The model under review builds one solid part; all positions refer to its coordinate system, in mm. A direction names the side the tool comes from. Round coordinates to 2 decimals unless told otherwise and drop trailing zeros. Write each loop counter-clockwise with the first axis right and the second up, starting at its lowest first coordinate (ties: lowest second). Pieces come first, ordered by that corner, then holes. Notation, with made-up numbers: M -26.75,21 L 12.25,21 A23 cw 12.25,41 Z; hole C 72.25,59.25 d5. An arc over 180 degrees is marked long. One line per item, written item: value. Start each with the question number.
1) Wall thickness on probe 1 along Y at (x, z) = (-6, 12); probe 2 along Z at (x, y) = (0, -1); probe 3 along Z at (x, y) = (0, 1.5): over which ranges is each line inside the solid? List them lowest first.
2) Tool access review of faces 4 (the face through (14.985, -2.218, -0.66)), 5 (the face through (2.2, 4.5, -11.2)): name each direction out of +Z, -Z, +X, -X, +Y, -Y from which nothing blocks a thin tool from reaching the whole face with its end or side.
3) For P1, Ø8, axis at y = -2.5, z = 5.5, coming from the +X side; P2, Ø4, axis at y = 7, z = 1.5, coming from the -X side; P3, Ø3, axis at y = 5.5, z = -6.5, coming from the -X side, all flat-tipped, find the tip position at first contact; note any pin that passes through.
4) Take a section at C-C, the plane z = 4. Write out the cut boundary in (x, y).
5) Take a section at D-D, the plane y = -1.5. Write out the cut boundary in (x, z), and give its area (3 significant figures).
6) Mouldability with a two-part tool opening along X and no side actions: class faces 1 (the face through (-2.2, 0, -11.2)), 2 (the face through (5.19, 2.22, 9.98)), 3 (the face through (0.65, 2.34, -1.01)) as +X half, -X half, draft (parallel to the pull), parting line (faces both ways), or undercut.
7) Take a section at A-A, the plane z = 0. Write out the cut boundary in (x, y).
8) Take a section at B-B, the plane x = 0. Write out the cut boundary in (y, z).
from build123d import *

# Parameters (mm, degrees)
SKETCH1_R            = 11.25
BOSS_EXTRUDE1_DEPTH  = 4.5
SKETCH2_R            = 15
BOSS_EXTRUDE2_DEPTH  = 4.5
SKETCH3_R            = 15
BOSS_EXTRUDE3_DEPTH  = 4.5
M2_CLEARANCE_HOLE1_D = 2.4


with BuildPart() as part:
    # Sketch1 → Boss-Extrude1 (new body)
    with BuildSketch(Plane(origin=(0, 0, 0), x_dir=(1, 0, 0), z_dir=(0, 1, 0))):
        Circle(SKETCH1_R)
    extrude(amount=BOSS_EXTRUDE1_DEPTH)

    # Sketch2 → Boss-Extrude2 (add)
    with BuildSketch(Plane(origin=(0, 4.5, 0), x_dir=(1, 0, 0), z_dir=(0, 1, 0))):
        Circle(SKETCH2_R)
    extrude(amount=BOSS_EXTRUDE2_DEPTH)

    # Sketch3 → Boss-Extrude3 (add)
    with BuildSketch(Plane(origin=(0, 0, 0), x_dir=(-1, 0, 0), z_dir=(0, -1, 0))):
        Circle(SKETCH3_R)
    extrude(amount=BOSS_EXTRUDE3_DEPTH)

    # M2 Clearance Hole1 (through all)
    with Locations(Plane(origin=(0, -4.5, 0), x_dir=(-1, 0, 0), z_dir=(0, -1, 0))):
        with Locations((0, 0)):
            Hole(M2_CLEARANCE_HOLE1_D / 2)


solid = part.part
Checked values:
1. probe 1: y = -4.5 to 0, 4.5 to 9
1. probe 2: z = -15 to -1.2, 1.2 to 15
1. probe 3: z = -11.25 to -1.2, 1.2 to 11.25
2. face 4: +Y, -Y
2. face 5: none
3. P1: stops at x = 14.92
3. P2: stops at x = -15
3. P3: stops at x = -14.14
4. outline: M -14.46,-4.5 L 14.46,-4.5 L 14.46,0 L 10.51,0 L 10.51,4.5 L 14.46,4.5 L 14.46,9 L -14.46,9 L -14.46,4.5 L -10.51,4.5 L -10.51,0 L -14.46,0 Z
5. outline: C 0,0 d30; hole C 0,0 d2.4
5. area: 702 mm2
6. face 1: draft
6. face 2: parting line
6. face 3: undercut
7. outline: M -15,-4.5 L -1.2,-4.5 L -1.2,9 L -15,9 L -15,4.5 L -11.25,4.5 L -11.25,0 L -15,0 Z; M 1.2,-4.5 L 15,-4.5 L 15,0 L 11.25,0 L 11.25,4.5 L 15,4.5 L 15,9 L 1.2,9 Z
8. outline: M -4.5,-15 L 0,-15 L 0,-11.25 L 4.5,-11.25 L 4.5,-15 L 9,-15 L 9,-1.2 L -4.5,-1.2 Z; M -4.5,1.2 L 9,1.2 L 9,15 L 4.5,15 L 4.5,11.25 L 0,11.25 L 0,15 L -4.5,15 Z
